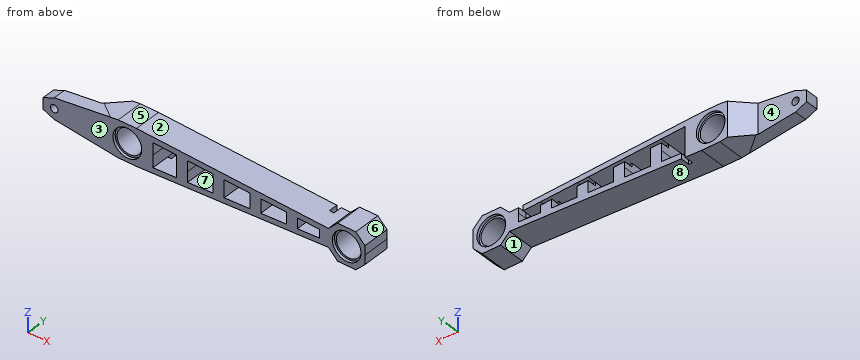
```python
from build123d import *
from OCP.BRepAlgoAPI import BRepAlgoAPI_Cut
from OCP.TopTools import TopTools_ListOfShape
from build123d.topology import SkipClean

# Parameters (mm, degrees)
SKETCH1_R           = 2.05
SKETCH1_R_2         = 6.85
BOSS_EXTRUDE1_DEPTH = 15
SKETCH1_3_R         = 7.85
CUT_EXTRUDE1_DEPTH  = 1.5
CUT_EXTRUDE2_START  = 13.5
SKETCH1_4_R         = 7.85
CUT_EXTRUDE2_DEPTH  = 1.5
CUT_EXTRUDE18_DEPTH = 15
CUT_EXTRUDE19_DEPTH = 15
CUT_EXTRUDE20_DEPTH = 5
CUT_EXTRUDE21_DEPTH = 25
BOSS_EXTRUDE2_START = 8
SKETCH9_R           = 2.05
BOSS_EXTRUDE2_DEPTH = 8
CUT_EXTRUDE22_DEPTH = 30


with BuildPart() as part:
    # Sketch1 → Boss-Extrude1 (new body)
    with BuildSketch(Plane(origin=(0, 0, 0), x_dir=(1, 0, 0), z_dir=(0, 1, 0))):
        Polygon((91.286914415, -0.000755057), (91.286914415, -5.000755057), (86.287669472, -10), (76.287669472, -10), (71.288424529, -5.000755057), (-33.712330528, -10), (-43.712330528, -10), (-78.712330528, -5.702540368), (-84.854022115, -3), (-84.854022115, 0), (-84.853996395, 3), (-78.712281638, 5.702487713), (-43.712244796, 9.999647278), (-33.712244796, 9.999561545), (71.288467397, 4.999416396), (76.2877552, 9.998618479), (86.287755199, 9.998532746), (91.286957282, 4.999244943), align=None)
        with Locations(Location((-78.712330528, 0, 0), (0, 0, 270))):
            Circle(SKETCH1_R, mode=Mode.SUBTRACT)
        with Locations(Location((81.287669472, 0, 0), (0, 0, 270))):
            Circle(SKETCH1_R_2, mode=Mode.SUBTRACT)
        with Locations(Location((-38.712330528, 0, 0), (0, 0, 270))):
            Circle(SKETCH1_R_2, mode=Mode.SUBTRACT)
    extrude(amount=BOSS_EXTRUDE1_DEPTH)

    # Sketch1<3> → Cut-Extrude1 (cut)
    with BuildSketch(Plane(origin=(0, 0, 0), x_dir=(1, 0, 0), z_dir=(0, 1, 0))):
        with Locations(Location((-38.712330528, 0, 0), (0, 0, 270))):
            Circle(SKETCH1_3_R)
        with Locations(Location((81.287669472, 0, 0), (0, 0, 270))):
            Circle(SKETCH1_3_R)
    extrude(amount=CUT_EXTRUDE1_DEPTH, mode=Mode.SUBTRACT)

    # Sketch1<4> → Cut-Extrude2 (cut)
    with BuildSketch(Plane(origin=(0, 0, 0), x_dir=(1, 0, 0), z_dir=(0, 1, 0)).offset(CUT_EXTRUDE2_START)):
        with Locations(Location((-38.712330528, 0, 0), (0, 0, 270))):
            Circle(SKETCH1_4_R)
        with Locations(Location((81.287669472, 0, 0), (0, 0, 270))):
            Circle(SKETCH1_4_R)
    extrude(amount=CUT_EXTRUDE2_DEPTH, mode=Mode.SUBTRACT)

    # Sketch2 → Cut-Extrude18 (cut)
    with BuildSketch(Plane(origin=(0, 15, 0), x_dir=(1, 0, 0), z_dir=(0, 1, 0))):
        Polygon((-24.712374044, 6.599650564), (-11.712369995, 5.985582494), (-11.712330529, -0.000306581), (-11.712330529, -5.986195656), (-24.712330529, -6.600349436), (-24.712330529, -0.000349436), align=None)
        Polygon((-5.712330529, -0.000286801), (-5.712368126, 5.702166462), (8.287636234, 5.040862387), (8.287669471, -0.000240649), (8.287669471, -5.041343686), (-5.712330529, -5.702740065), align=None)
    extrude(amount=-CUT_EXTRUDE18_DEPTH, mode=Mode.SUBTRACT)

    # Sketch5 → Cut-Extrude19 (cut)
    with BuildSketch(Plane(origin=(0, 15, 0), x_dir=(1, 0, 0), z_dir=(0, 1, 0))):
        Polygon((14.287669471, -4.757888095), (14.287638103, 4.757446355), (28.287642463, 4.09614228), (28.287669471, -4.096491716), align=None)
        Polygon((34.287644332, 3.812726248), (48.287648692, 3.151422173), (48.287669471, -3.151639747), (34.287669471, -3.813036126), align=None)
        Polygon((54.287650561, 2.868006141), (66.2876543, 2.301174077), (66.287669472, -2.301272974), (54.287669471, -2.868184156), align=None)
    extrude(amount=-CUT_EXTRUDE19_DEPTH, mode=Mode.SUBTRACT)


with BuildPart() as cut_extrude20_tool:
    # Sketch6 → Cut-Extrude20 (new body)
    with BuildSketch(Plane(origin=(0, 15, 0), x_dir=(1, 0, 0), z_dir=(0, 1, 0))):
        Polygon((-24.712374044, 9.570986737), (-22.664694465, 9.473476016), (-22.664694465, 6.50292639), (-24.712374044, 6.599650564), align=None)
        Polygon((64.239989057, -2.398010718), (66.287669472, -2.301272974), (66.287669472, -5.238848578), (64.239989057, -5.336341743), (63.843088459, -5.355238781), (63.843088459, -2.416761333), align=None)
        Polygon((54.287669471, -1.068184156), (54.287669471, -2.868184156), (48.287669471, -3.151639747), (48.287669471, -1.575940198), (48.294422194, -1.333159375), align=None)
        Polygon((34.287669471, -1.952430065), (28.287669471, -2.217703838), (28.287669471, -4.096491716), (34.287669471, -3.813036126), align=None)
        Polygon((8.287669471, -3.101949747), (14.287669471, -2.836675974), (14.287669471, -4.757888095), (8.287669471, -5.041343686), align=None)
        Polygon((-5.712330529, -3.720921883), (-11.712330529, -3.986195656), (-11.712330529, -5.986195656), (-5.712330529, -5.702740065), align=None)
    extrude(amount=-CUT_EXTRUDE20_DEPTH)


with BuildPart() as part_1:
    add(part.part)

    # Cut-Extrude20: cut by cut_extrude20_tool, with a tolerance
    cut_extrude20_stock = TopTools_ListOfShape()
    cut_extrude20_stock.Append(part_1.part.wrapped)
    cut_extrude20_tools = TopTools_ListOfShape()
    cut_extrude20_tools.Append(cut_extrude20_tool.part.wrapped)
    cut_extrude20_cut = BRepAlgoAPI_Cut()
    cut_extrude20_cut.SetArguments(cut_extrude20_stock)
    cut_extrude20_cut.SetTools(cut_extrude20_tools)
    cut_extrude20_cut.SetFuzzyValue(0.00001)
    cut_extrude20_cut.Build()
    add(Compound.cast(cut_extrude20_cut.Shape()).solids(), mode=Mode.REPLACE)

    # Sketch8 → Cut-Extrude21 (cut)
    with BuildSketch(Plane.XY.offset(10)):
        Polygon((-47.904022115, 0), (-58.104022115, 8), (-84.854022115, 8), (-84.854022115, 0), align=None)
    extrude(amount=-CUT_EXTRUDE21_DEPTH, mode=Mode.SUBTRACT)

    # Sketch9 → Boss-Extrude2 (add)
    with SkipClean():  # the faces are left unmerged after this step: merging them gives an invalid solid
        with BuildSketch(Plane.XZ.offset(-8).offset(BOSS_EXTRUDE2_START)):
            Polygon((-84.854022115, 3), (-84.853996395, -3), (-78.712281638, -5.702487713), (-47.032796515, -9.591963691), (-47.380824321, 9.5495656), (-78.712330528, 5.702540368), align=None)
            with Locations((-78.712330528, 0)):
                Circle(SKETCH9_R, mode=Mode.SUBTRACT)
        extrude(amount=-BOSS_EXTRUDE2_DEPTH)

    # Sketch10 → Cut-Extrude22 (cut)
    with BuildSketch(Plane(origin=(8.5727e-05, 0, -9.999272518), x_dir=(-0.9999999999632491, 0, -8.573327994754198e-06), z_dir=(8.573327994754198e-06, 0, -0.9999999999632491))):
        Polygon((47.904022112, 15), (58.104022112, 7), (84.854022112, 7), (84.854022112, 15), align=None)
    extrude(amount=-CUT_EXTRUDE22_DEPTH, mode=Mode.SUBTRACT)


solid = part_1.part
```
Check sheet for the modelled part. Datum: model origin and axes. Units: mm. Face numbers are marked on the shaded views. A direction names the side the tool comes from. Coordinates: 2 decimals unless noted, no trailing zeros. Write each loop counter-clockwise with the first axis right and the second up, starting at its lowest first coordinate (ties: lowest second). Pieces come first, ordered by that corner, then holes. Notation, with made-up numbers: M -9.75,21 L 24.25,21 A20 cw 24.25,36 Z; hole C -34,37.5 d1. An arc over 180 degrees is marked long. Use one line per item in the form item = value.
Item 1: Release check for a two-part mould opening along X. For the marked faces 5, 6, 7 and 8 record: pulls with the +X half, pulls with the -X half, needs draft (parallel to the pull), parting line crosses it, or undercut.
Answer below:
face_5 = needs draft
face_6 = pulls with the +X half
face_7 = undercut
face_8 = undercut
Item 2: Material ranges on L1, parallel to X at y = 4, z = -4; L2, parallel to Z at x = 60, y = 6; L3, parallel to Z at x = -36, y = 14, recorded low to high. Write a range as from..to.
Answer below:
L1 = -82.58..-44.27, -33.15..-24.71, -11.71..-5.71, 8.29..14.29, 28.29..75.73, 86.85..91.29
L2 = -5.54..-2.6, 2.6..5.54
L3 = -10..-7.37, 7.37..10
Item 3: Gauge pin test, flat ends, axial feed: pin 1 Ø1.8 at (y, z) = (9.5, 3.5) entering from -X; pin 2 Ø4 at (x, z) = (16, 3) entering from +Y; pin 3 Ø2.5 at (y, z) = (12.5, 3.5) entering from -X; pin 4 Ø1.5 at (y, z) = (13.5, -7.5) entering from +X. Record the tip position at first contact, or that the pin passes through.
Answer below:
pin_1 = -56.06
pin_2 = 15
pin_3 = -52.69
pin_4 = 89.54
Item 4: Sectioned sample at A-A, the plane x = 38. Record the cut outline in (y, z), and give its area (3 significant figures).
Answer below:
outline = M 0,-6.58 L 15,-6.58 L 15,-3.64 L 0,-3.64 Z; M 0,3.64 L 15,3.64 L 15,6.59 L 0,6.59 Z
area = 88.4 mm^2
Item 5: Set-up check for the marked faces 1, 2, 3 and 4: record each of +Z, -Z, +X, -X, +Y, -Y from which the full face is reachable in a straight line by a thin tool's end or side.
Answer below:
face_1 = -Z, +Y, -Y
face_2 = +Z, +Y, -Y
face_3 = +Z, -Z, +X, -X, -Y
face_4 = +Z, -Z, -X, +Y
Item 6: Sectioned sample at B-B, the plane x = -17.5. Record the cut outline in (y, z).
Answer below:
outline = M 0,-9.23 L 15,-9.23 L 15,-6.26 L 0,-6.26 Z; M 0,6.26 L 15,6.26 L 15,9.23 L 0,9.23 Z
